from build123d import *

# Parameters (mm, degrees)
SKETCH1_R             = 52.3875
SKETCH1_R_2           = 23.5
BOSS_EXTRUDE1_DEPTH   = 11.43
M6_CLEARANCE_HOLE1_D  = 6.6
F_5_0MM_DOWEL_HOLE1_D = 5
CIRPATTERN1_COUNT     = 4


with BuildPart() as part:
    # Sketch1 → Boss-Extrude1 (new body)
    with BuildSketch(Plane(origin=(0, 0, 0), x_dir=(1, 0, 0), z_dir=(0, 1, 0))):
        Polygon((-234.329030184, -12.7), (113.061428613, -12.7), (113.061428613, -187.604888893), (-213.064788009, -187.65872147), align=None)
        with Locations(Location((-123.19, -116.001477372, 0), (0, 0, 270))):
            Circle(SKETCH1_R, mode=Mode.SUBTRACT)
        with Locations(Location((54.61, -127, 0), (0, 0, 270))):
            Circle(SKETCH1_R_2, mode=Mode.SUBTRACT)
    extrude(amount=BOSS_EXTRUDE1_DEPTH)

    # M6 Clearance Hole1 (through all)
    with Locations(Plane(origin=(0, 0, 0), x_dir=(-1, 0, 0), z_dir=(0, -1, 0))):
        with Locations((-10.033704867, -23.334197365), (211.518182886, -18.798178744), (205.575185514, -154.375359311)):
            Hole(M6_CLEARANCE_HOLE1_D / 2)

    # Ø5.0mm Dowel Hole1 (through all)
    with Locations(Plane(origin=(0, 0, 0), x_dir=(-1, 0, 0), z_dir=(0, -1, 0))):
        with Locations((123.19, -173.151477372)):
            f_5_0mm_dowel_hole1 = Hole(F_5_0MM_DOWEL_HOLE1_D / 2)

    # CirPattern1: Ø5.0mm Dowel Hole1 ×4 about axis
    cirpattern1_axis = Axis((-123.19, 0, 116.001477372), (0, 1, 0))
    for i in range(1, CIRPATTERN1_COUNT):
        add(f_5_0mm_dowel_hole1.rotate(cirpattern1_axis, i * 360 / CIRPATTERN1_COUNT), mode=Mode.SUBTRACT)


solid = part.part
Geometry check sheet. Reference: the model listing, model coordinates, mm. Coordinates: 2 decimals unless noted, no trailing zeros. Order: outer loops, then holes, each group sorted by start corner. A loop starts at its lowest first (then second) coordinate and runs counter-clockwise, first axis right, second up. Notation, with made-up numbers: M -6,15 L 49,15 A28 ccw 49,39 Z; hole C 37.5,41 d10. An arc over 180 degrees is marked long. Use CSV: the item, a comma, the result in double quotes.
Item 1: Mould release check, pull along X, two halves, no side actions. Record for faces 1 (the cylindrical face through (-213.95, 5.8, 16.57)), 2 (the flat face through (113.061, 6, 99)), 3 (the flat face through (-58, 0, 99)), 4 (the cylindrical face through (13.18, 5.8, 22.34)): pulls with the +X half, pulls with the -X half, needs draft (parallel to the pull), parting line crosses it, or undercut.
Returned:
face 1,"undercut"
face 2,"pulls with the +X half"
face 3,"needs draft"
face 4,"undercut"
Item 2: Thickness scan on line 1 along X through (y, z) = (2, 139); line 2 along Z through (x, y) = (-212, 8); line 3 along Z through (x, y) = (-141.5, 1.25). Record the ranges inside material, lowest first.
Returned:
line 1,"x = -218.98 to -170.26, -76.12 to 34.4, 74.82 to 113.06"
line 2,"z = 12.7 to 15.53, 22.06 to 187.66"
line 3,"z = 12.7 to 66.92, 165.09 to 187.65"
Item 3: Cross-section at B-B on z = 127. Record the cut outline in (x, y), then the cut area to 3 significant figures.
Returned:
outline,"M -220.44,0 L -174.41,0 L -174.41,11.43 L -220.44,11.43 Z; M -71.97,0 L 31.11,0 L 31.11,11.43 L -71.97,11.43 Z; M 78.11,0 L 113.06,0 L 113.06,11.43 L 78.11,11.43 Z"
area,"2,100 mm2"
Item 4: Cross-section at A-A on x = 54.61. Record the cut outline in (y, z).
Returned:
outline,"M 0,12.7 L 11.43,12.7 L 11.43,103.5 L 0,103.5 Z; M 0,150.5 L 11.43,150.5 L 11.43,187.61 L 0,187.61 Z"
Item 5: Gauge pin test, flat ends, axial feed: pin 1 Ø6.5 at (x, z) = (-123.19, 173.15) entering from +Y; pin 2 Ø4 at (x, y) = (-178.5, 5) entering from +Z; pin 3 Ø6 at (x, y) = (-80, 4.5) entering from +Z. Record the tip position at first contact, or that the pin passes through.
Returned:
pin 1,"stops at y = 11.43"
pin 2,"stops at z = 187.65"
pin 3,"stops at z = 187.64"
Item 6: Cross-section at C-C on y = 1.75. Give the number of separate pieces and of enclosed holes in the cut face, then the cut area to 3 significant figures.
Returned:
separate pieces,"1"
enclosed holes,"9"
area,"48,400 mm2"
